For this review, take the finished solid that the model builds, in its own axes (mm). A direction names the side the tool comes from. Give positions to 0.01 mm unless a question says otherwise; leave off trailing zeros. Write each loop counter-clockwise with the first axis right and the second up, starting at its lowest first coordinate (ties: lowest second). Pieces come first, ordered by that corner, then holes.
1) We need section A-A on x = 0. Give the boundary of the cut face in (y, z) (3 decimals), and give its area (4 significant figures).
2) Draft analysis for pull direction Z (two halves, no side actions). For faces 4 (the face through (3, -11, -10)), 5 (the face through (9, 7, 0)), 6 (the face through (-6.34, 12.2, -4.49)), state which applies: pulls with the +Z half, pulls with the -Z half, needs draft (parallel to the pull), parting line crosses it, or undercut.
3) We need section C-C on z = -7. Give the boundary of the cut face in (x, y) (3 decimals).
4) For P1, Ø1.5, axis at y = 1, z = -4.5, coming from the +X side; P2, Ø5, axis at x = 1, z = -6.5, coming from the +Y side (3 decimals); P3, Ø4, axis at x = 2.5, z = -2, coming from the +Y side; P4, Ø3, axis at x = -7.5, y = -3.5, coming from the +Z side, all flat-tipped, find the tip position at first contact; note any pin that passes through.
5) Wall thickness on line 1 along Y through (x, z) = (0, -6.75) (3 decimals); line 2 along Y through (x, z) = (0, -3.5); line 3 along Z through (x, y) = (9, -10.5): over which ranges is each line inside the solid? List them lowest first.
6) Machinability: for faces 1 (the face through (-13, -5, -4)), 2 (the face through (1.445, -11.006, -5.07)), 3 (the face through (3.09, 13.91, -1.97)), which of the approach directions +Z, -Z, +X, -X, +Y, -Y give a long, thin tool a straight path to every point of the face, cutting with its end or side? Answer none if there is none.
7) We need section D-D on x = -11.5. Give the boundary of the cut face in (y, z).
from build123d import *


with BuildPart() as part:
    # 草图1 → 旋转1 (revolve)
    with BuildSketch(Plane(origin=(0, 0, 0), x_dir=(1, 0, 0), z_dir=(0, 1, 0)), mode=Mode.PRIVATE) as revolve_1_sk:
        Polygon((11.1, 0), (11.1, 10), (15.875, 10), (15.875, 5), (13.75, 5), (13.75, 4), (14.25, 4), (14.25, 0), align=None)
    revolve(revolve_1_sk.sketch.rotate(Axis((0, 0, -19.14057971), (0, 0, 1)), 180), axis=Axis((0, 0, -19.14057971), (0, 0, 1)))  # turned: the seam where the file's is


solid = part.part
Results list:
1. outline: (-15.875, -10) - (-11.1, -10) - (-11.1, 0) - (-14.25, 0) - (-14.25, -4) - (-13.75, -4) - (-13.75, -5) - (-15.875, -5) - close; (11.1, -10) - (15.875, -10) - (15.875, -5) - (13.75, -5) - (13.75, -4) - (14.25, -4) - (14.25, 0) - (11.1, 0) - close
1. area: 78.25 mm2
2. face 4: pulls with the -Z half
2. face 5: pulls with the +Z half
2. face 6: undercut
3. outline: circle Ø31.75 at (0, 0); hole circle Ø22.2 at (0, 0)
4. P1: stops at x = 15.87
4. P2: stops at y = 15.875
4. P3: stops at y = 14.24
4. P4: passes through
5. line 1: y = -15.875 to -11.1, 11.1 to 15.875
5. line 2: y = -14.25 to -11.1, 11.1 to 14.25
5. line 3: z = -10 to -5, -4 to 0
6. face 1: none
6. face 2: +Z, -Z
6. face 3: +Z
7. outline: (-10.94, -10) - (10.94, -10) - (10.94, -5) - (7.54, -5) - (7.54, -4) - (8.42, -4) - (8.42, 0) - (-8.42, 0) - (-8.42, -4) - (-7.54, -4) - (-7.54, -5) - (-10.94, -5) - close
